from build123d import *

# Parameters (mm, degrees)
DODANIE_WYCI_GNI_CIE1_DEPTH = 5
DODANIE_WYCI_GNI_CIE2_DEPTH = 9
SZKIC4_R                    = 1.45
WYTNIJ_WYCI_GNI_CIE1_DEPTH  = 6
SZKIC3_R                    = 3
DODANIE_WYCI_GNI_CIE3_DEPTH = 5


with BuildPart() as part:
    # Szkic1 → Dodanie-wyciągnięcie1 (new body)
    with BuildSketch(Plane(origin=(0, 0, 0), x_dir=(1, 0, 0), z_dir=(0, 1, 0))):
        Polygon((24, 4.5), (27.122498999, 2), (27.122498999, -2), (24, -4.5), (-24, -4.5), (-28, -2), (-28, 2), (-24, 4.5), align=None)
    extrude(amount=DODANIE_WYCI_GNI_CIE1_DEPTH)

    # Szkic2 → Dodanie-wyciągnięcie2 (add)
    with BuildSketch(Plane.XY.offset(4.5)):
        with BuildLine():
            Line((-7.5, 5), (7.5, 5))
            Line((7.5, 5), (7.5, 10.25))
            ThreePointArc((7.5, 10.25), (0, 17.75), (-7.5, 10.25))
            Line((-7.5, 10.25), (-7.5, 5))
        make_face()
    extrude(amount=-DODANIE_WYCI_GNI_CIE2_DEPTH)

    # Szkic4 → Wytnij-wyciągnięcie1 (cut)
    with BuildSketch(Plane(origin=(0, 5, 0), x_dir=(1, 0, 0), z_dir=(0, 1, 0))):
        with Locations(Location((12.40562475, 0, 0), (0, 0, 270))):
            Circle(SZKIC4_R)
        with Locations(Location((21.90562475, 0, 0), (0, 0, 270))):
            Circle(SZKIC4_R)
        with Locations(Location((-12.57201541, 0.053033314, 0), (0, 0, 270))):
            Circle(SZKIC4_R)
        with Locations(Location((-22.71604623, 0.159099943, 0), (0, 0, 270))):
            Circle(SZKIC4_R)
    extrude(amount=-WYTNIJ_WYCI_GNI_CIE1_DEPTH, mode=Mode.SUBTRACT)

    # Szkic3 → Dodanie-wyciągnięcie3 (add)
    with BuildSketch(Plane.XY.offset(4.5)):
        with Locations(Location((0, 11, 0), (0, 0, 180))):
            Circle(SZKIC3_R)
    extrude(amount=DODANIE_WYCI_GNI_CIE3_DEPTH)


solid = part.part
Source: CAD feature listing. Evaluate the final solid. Frame: model axes, mm. A direction names the side the tool comes from. Give positions to 0.01 mm unless a question says otherwise; leave off trailing zeros. Order: outer loops, then holes, each group sorted by start corner. A loop starts at its lowest first (then second) coordinate and runs counter-clockwise, first axis right, second up. Notation, with made-up numbers: (11.5, -17.5) -> (67.5, -17.5) arc R16 ccw to (67.5, 8.5) -> close; hole circle Ø5 at (-15, 11.5). An arc over 180 degrees is marked (long way). Write item = value, one per line.
Q1. Pin query (flat end, axial travel): pin 1 (1.6 mm diameter, centred on y = 8, z = -1, fed in from -X); pin 2 (1.5 mm diameter, centred on y = 11, z = 6, fed in from -X); pin 3 (3 mm diameter, centred on y = 14.5, z = -1.5, fed in from +X). Return the tip coordinate at first contact, or that it passes through.
Data:
pin_1 = -7.5
pin_2 = -3
pin_3 = 6.98
Q2. Cut plane D-D, the plane y = 11. Output: boundary loops of the cut face in (x, z).
Data:
outline = (-7.46, -4.5) -> (7.46, -4.5) -> (7.46, 4.5) -> (3, 4.5) -> (3, 9.5) -> (-3, 9.5) -> (-3, 4.5) -> (-7.46, 4.5) -> close
Q3. Cut plane C-C, the plane y = 2.75. Output: boundary loops of the cut face in (x, z).
Data:
outline = (-28, -2) -> (-24, -4.5) -> (24, -4.5) -> (27.12, -2) -> (27.12, 2) -> (24, 4.5) -> (-24, 4.5) -> (-28, 2) -> close; hole circle Ø2.9 at (-22.72, -0.16); hole circle Ø2.9 at (-12.57, -0.05); hole circle Ø2.9 at (12.41, 0); hole circle Ø2.9 at (21.91, 0)
Q4. Cut plane A-A, the plane x = 0. Output: boundary loops of the cut face in (y, z), and give its area (3 significant figures).
Data:
outline = (0, -4.5) -> (17.75, -4.5) -> (17.75, 4.5) -> (14, 4.5) -> (14, 9.5) -> (8, 9.5) -> (8, 4.5) -> (0, 4.5) -> close
area = 190 mm^2
Q5. Cut plane B-B, the plane z = -0.5. Output: boundary loops of the cut face in (x, y), and give its area (3 significant figures).
Data:
outline = (-28, 0) -> (-24.13, 0) -> (-24.13, 5) -> (-28, 5) -> close; (-21.31, 0) -> (-13.95, 0) -> (-13.95, 5) -> (-21.31, 5) -> close; (-11.19, 0) -> (11.04, 0) -> (11.04, 5) -> (7.5, 5) -> (7.5, 10.25) arc R7.5 ccw to (-7.5, 10.25) -> (-7.5, 5) -> (-11.19, 5) -> close; (13.77, 0) -> (20.54, 0) -> (20.54, 5) -> (13.77, 5) -> close; (23.27, 0) -> (27.12, 0) -> (27.12, 5) -> (23.27, 5) -> close
area = 388 mm^2
Q6. Set-up query: faces 1 (the face through (7.5, 8, 0)), 2 (the face through (-2.86, 10.1, 6.96)), 3 (the face through (-7.5, 8, 0)). Return all of +Z, -Z, +X, -X, +Y, -Y with unobstructed straight access to the full face (end or side cutting, diameter ignored); none if empty.
Data:
face_1 = +Z, -Z, +X, +Y
face_2 = +Z
face_3 = +Z, -Z, -X, +Y
Q7. Pull-direction query (Z, two-part tool) for faces 4 (the face through (-13.988, 2.535, -0.367)), 5 (the face through (25.5, 2.5, -3.3)), 6 (the face through (17, 5, 0)); classes: released by +Z, released by -Z, zero draft, split by the parting line, or undercut.
Data:
face_4 = undercut
face_5 = released by -Z
face_6 = zero draft
Q8. Material intervals for line 1 (X direction, y = 2.3, z = 0); line 2 (X direction, y = 4, z = 0.25); line 3 (Z direction, x = 0.5, y = 2.75), sorted ascending. Write a range as from..to.
Data:
line_1 = -28..-24.16, -21.27..-14.02, -11.12..10.96, 13.86..20.46, 23.36..27.12
line_2 = -28..-24.11, -21.32..-13.99, -11.15..10.98, 13.83..20.48, 23.33..27.12
line_3 = -4.5..4.5
